The listing builds one solid part. Answer for the finished solid, in the listing's coordinates (mm). Round coordinates to 2 decimals unless told otherwise and drop trailing zeros. Loops run counter-clockwise (first coordinate to the right, second up) from the corner with the lowest first, then second, coordinate; pieces in that order, holes last. Notation, with made-up numbers: M 20,43.5 L 24,43.5 A19 cw 24,71.5 Z; hole C 42,-31 d11. An arc over 180 degrees is marked long. Answer as a JSON object with one key per item and string values.
```python
from build123d import *

# Parameters (mm, degrees)
F1_DEPTH = 3.4
F2_START = 0.6
F2_DEPTH = 2.2


with BuildPart() as f1:
    # F0 (on Top) → F1 (new body)
    with BuildSketch(Plane.XY):
        Polygon((22.546146065, 22.093931213), (3.5531178582, 0), (4.1273287497, 0), (22.2029884881, 21.0267882794), align=None)
        Polygon((22.2029884881, 21.0267882794), (4.1273287497, 0), (48.128593713, 0), (48.128593713, 21.0267882794), align=None)
        Polygon((3.5531178582, 0), (-12.671406287, 0), (-12.671406287, -2.7), (47.9993857443, -2.7), (48.128593713, 0), (4.1273287497, 0), align=None)
    extrude(amount=F1_DEPTH)

    # F0 (on Top) → F2 (cut)
    with BuildSketch(Plane.XY.offset(F2_START)):
        Polygon((22.2029884881, 21.0267882794), (4.1273287497, 0), (48.128593713, 0), (48.128593713, 21.0267882794), align=None)
        Polygon((48.128593713, 22.093931213), (22.546146065, 22.093931213), (22.2029884881, 21.0267882794), (48.128593713, 21.0267882794), align=None)
    extrude(amount=F2_DEPTH, mode=Mode.SUBTRACT)


solid = f1.part
```
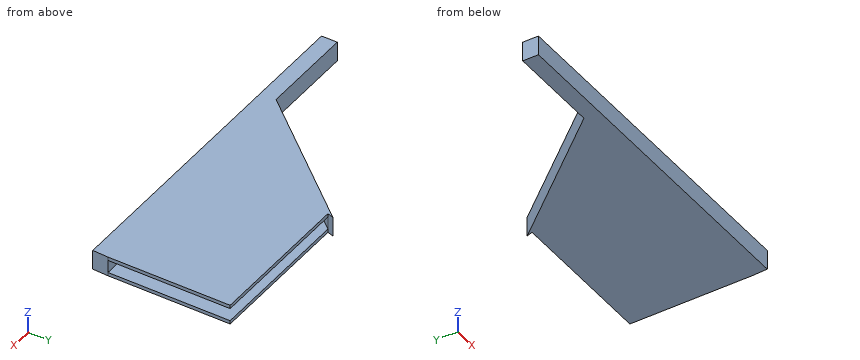
Item 1: Flat-ended cylindrical pins translate along their axes: P1, Ø1.1, axis at x = 26, z = 1.5, coming from the +Y side; P2, Ø0.7, axis at x = 36, z = 0.5, coming from the +Y side. Find the tip coordinate at first contact, or state that the pin passes through.
Values follow:
{"P1": "y = 0", "P2": "y = 21.03"}
Item 2: The part is cut by section B-B (z = 1.15). Give the vertices of the cut face in (x, y), then the cut area to 3 significant figures.
Values follow:
{"outline": "M -12.67,-2.7 L 48,-2.7 L 48.13,0 L 4.13,0 L 22.2,21.03 L 22.55,22.09 L 3.55,0 L -12.67,0 Z", "area": "176 mm^2"}
Item 3: The part is cut by section D-D (x = 13.5). Give the vertices of the cut face in (y, z).
Values follow:
{"outline": "M -2.7,0 L 11.57,0 L 11.57,3.4 L -2.7,3.4 Z; hole M 0,0.6 L 10.9,0.6 L 10.9,2.8 L 0,2.8 Z"}
Item 4: Straight lines are drawn through the part: line 1 (Z direction, x = 31.5, y = 0.25); line 2 (Y direction, x = -0.5, z = 3.1); line 3 (Y direction, x = 14.5, z = 1.2). For each, find the intervals that lie inside material, in ascending order.
Values follow:
{"line 1": "0 to 0.6, 2.8 to 3.4", "line 2": "-2.7 to 0", "line 3": "-2.7 to 0, 12.07 to 12.73"}
Item 5: The part is cut by section C-C (y = 17). Give the vertices of the cut face in (x, z), then the cut area to 3 significant figures.
Values follow:
{"outline": "M 18.17,0 L 48.13,0 L 48.13,0.6 L 18.74,0.6 L 18.74,2.8 L 48.13,2.8 L 48.13,3.4 L 18.17,3.4 Z", "area": "37.2 mm^2"}
Item 6: The part is cut by section A-A (x = 21.5). Give the vertices of the cut face in (y, z).
Values follow:
{"outline": "M -2.7,0 L 20.88,0 L 20.88,3.4 L -2.7,3.4 Z; hole M 0,0.6 L 20.21,0.6 L 20.21,2.8 L 0,2.8 Z"}
